from build123d import *

# Parameters (mm, degrees)
SKETCH1_W           = 72
SKETCH1_H           = 47
BOSS_EXTRUDE1_DEPTH = 4
SKETCH3_W           = 72
SKETCH3_H           = 47
SKETCH3_W_2         = 67
SKETCH3_H_2         = 42
BOSS_EXTRUDE3_DEPTH = 32
SKETCH2_R           = 0.9
BOSS_EXTRUDE4_DEPTH = 16
SKETCH4_R           = 2
BOSS_EXTRUDE5_DEPTH = 6
SKETCH5_W           = 12
SKETCH5_H           = 8
CUT_EXTRUDE1_DEPTH  = 6
FILLET2_R           = 2
FILLET3_R           = 2
SKETCH11_W          = 24
SKETCH11_H          = 20
BOSS_EXTRUDE7_DEPTH = 20
SKETCH12_W          = 20
SKETCH12_H          = 16
CUT_EXTRUDE4_DEPTH  = 20
SKETCH13_W          = 15
SKETCH13_H          = 9
CUT_EXTRUDE5_DEPTH  = 20
FILLET4_R           = 2
FILLET5_R           = 2
SKETCH14_W          = 6
SKETCH14_H          = 25
CUT_EXTRUDE6_DEPTH  = 5
FILLET6_R           = 2
SKETCH15_W          = 68
SKETCH15_H          = 6
BOSS_EXTRUDE8_DEPTH = 25
FILLET7_R           = 5
CUT_EXTRUDE7_DEPTH  = 25


with BuildPart() as part:
    # Sketch1 → Boss-Extrude1 (new body)
    with BuildSketch(Plane(origin=(0, 0, 0), x_dir=(1, 0, 0), z_dir=(0, 1, 0))):
        with Locations((25.5, 13)):
            Rectangle(SKETCH1_W, SKETCH1_H)
    extrude(amount=BOSS_EXTRUDE1_DEPTH)

    # Sketch3 → Boss-Extrude3 (add)
    with BuildSketch(Plane(origin=(0, 4, 0), x_dir=(1, 0, 0), z_dir=(0, 1, 0))):
        with Locations((25.5, 13)):
            Rectangle(SKETCH3_W, SKETCH3_H)
        with Locations((25.5, 13)):
            Rectangle(SKETCH3_W_2, SKETCH3_H_2, mode=Mode.SUBTRACT)
    extrude(amount=BOSS_EXTRUDE3_DEPTH)

    # Sketch2 → Boss-Extrude4 (add)
    with BuildSketch(Plane(origin=(0, 4, 0), x_dir=(1, 0, 0), z_dir=(0, 1, 0))):
        with Locations(Location((-1.2, 27.2, 0), (0, 0, 270))):
            Circle(SKETCH2_R)
        with Locations(Location((-1.2, -1.2, 0), (0, 0, 90))):
            Circle(SKETCH2_R)
        with Locations(Location((52.2, -1.2, 0), (0, 0, 270))):
            Circle(SKETCH2_R)
        with Locations(Location((52.2, 27.2, 0), (0, 0, 90))):
            Circle(SKETCH2_R)
    extrude(amount=BOSS_EXTRUDE4_DEPTH)

    # Sketch4 → Boss-Extrude5 (add)
    with BuildSketch(Plane(origin=(0, 4, 0), x_dir=(1, 0, 0), z_dir=(0, 1, 0))):
        with Locations(Location((-1.2, 27.2, 0), (0, 0, 270))):
            Circle(SKETCH4_R)
        with Locations(Location((-1.2, -1.2, 0), (0, 0, 90))):
            Circle(SKETCH4_R)
        with Locations(Location((52.2, -1.2, 0), (0, 0, 270))):
            Circle(SKETCH4_R)
        with Locations(Location((52.2, 27.2, 0), (0, 0, 90))):
            Circle(SKETCH4_R)
    extrude(amount=BOSS_EXTRUDE5_DEPTH)

    # Sketch5 → Cut-Extrude1 (cut)
    with BuildSketch(Plane(origin=(61.5, 0, 0), x_dir=(0, 0, -1), z_dir=(1, 0, 0))):
        with Locations((10, 16)):
            Rectangle(SKETCH5_W, SKETCH5_H)
    extrude(amount=-CUT_EXTRUDE1_DEPTH, mode=Mode.SUBTRACT)

    # Fillet2
    fillet2_edges = [part.edges().sort_by_distance(p)[0] for p in [
        (-10.5, 18, 10.5),
        (-10.5, 18, -36.5),
        (61.5, 18, -36.5),
        (61.5, 18, 10.5),
    ]]
    fillet(fillet2_edges, radius=FILLET2_R)

    # Fillet3
    fillet3_edges = [part.edges().sort_by_distance(p)[0] for p in [
        (60.25, 20, -4),
        (60.25, 20, -16),
    ]]
    fillet(fillet3_edges, radius=FILLET3_R)

    # Sketch11 → Boss-Extrude7 (add)
    with BuildSketch(Plane.ZY.offset(10.5)):
        with Locations((-15.5, 24)):
            Rectangle(SKETCH11_W, SKETCH11_H)
    extrude(amount=BOSS_EXTRUDE7_DEPTH)

    # Sketch12 → Cut-Extrude4 (cut)
    with BuildSketch(Plane(origin=(-8, 0, 0), x_dir=(0, 0, -1), z_dir=(1, 0, 0))):
        with Locations((15.5, 24)):
            Rectangle(SKETCH12_W, SKETCH12_H)
    extrude(amount=-CUT_EXTRUDE4_DEPTH, mode=Mode.SUBTRACT)

    # Sketch13 → Cut-Extrude5 (cut)
    with BuildSketch(Plane.ZY.offset(30.5)):
        with Locations((-15.5, 24)):
            Rectangle(SKETCH13_W, SKETCH13_H)
    extrude(amount=-CUT_EXTRUDE5_DEPTH, mode=Mode.SUBTRACT)

    # Fillet4
    fillet4_edges = [part.edges().sort_by_distance(p)[0] for p in [
        (-18, 16, -25.5),
        (-18, 16, -5.5),
        (-18, 32, -5.5),
        (-18, 32, -25.5),
    ]]
    fillet(fillet4_edges, radius=FILLET4_R)

    # Fillet5
    fillet5_edges = [part.edges().sort_by_distance(p)[0] for p in [
        (-20.5, 34, -27.5),
        (-20.5, 14, -27.5),
        (-20.5, 14, -3.5),
        (-20.5, 34, -3.5),
    ]]
    fillet(fillet5_edges, radius=FILLET5_R)

    # Sketch14 → Cut-Extrude6 (cut)
    with BuildSketch(Plane.ZY.offset(10.5)):
        with Locations((3, 24.5)):
            Rectangle(SKETCH14_W, SKETCH14_H)
    extrude(amount=-CUT_EXTRUDE6_DEPTH, mode=Mode.SUBTRACT)

    # Fillet6
    fillet6_edges = [part.edges().sort_by_distance(p)[0] for p in [
        (-9.25, 12, 0),
        (-9.25, 12, 6),
    ]]
    fillet(fillet6_edges, radius=FILLET6_R)

    # Sketch15 → Boss-Extrude8 (add)
    with BuildSketch(Plane.XY.offset(10.5)):
        with Locations((25.5, 3)):
            Rectangle(SKETCH15_W, SKETCH15_H)
    extrude(amount=BOSS_EXTRUDE8_DEPTH)

    # Fillet7
    fillet7_edges = [part.edges().sort_by_distance(p)[0] for p in [
        (-8.5, 3, 35.5),
        (59.5, 3, 35.5),
    ]]
    fillet(fillet7_edges, radius=FILLET7_R)

    # Sketch16 → Cut-Extrude7 (cut)
    with BuildSketch(Plane(origin=(0, 6, 0), x_dir=(1, 0, 0), z_dir=(0, 1, 0))):
        with BuildLine():
            Line((5.870048695, -18.078882232), (45.129951305, -18.078882232))
            ThreePointArc((45.129951305, -18.078882232), (49.279951305, -22.228882232), (45.129951305, -26.378882232))
            Line((45.129951305, -26.378882232), (5.870048695, -26.378882232))
            ThreePointArc((5.870048695, -26.378882232), (1.720048695, -22.228882232), (5.870048695, -18.078882232))
        make_face()
    extrude(amount=-CUT_EXTRUDE7_DEPTH, mode=Mode.SUBTRACT)


solid = part.part
Could you check a few things on this model? Use its own coordinates, in mm. A direction names the side the tool comes from. Coordinates: 2 decimals unless noted, no trailing zeros. Order: outer loops, then holes, each group sorted by start corner. A loop starts at its lowest first (then second) coordinate and runs counter-clockwise, first axis right, second up.
Q1. Suppose I cut it at C-C on x = 25. Please give me the cut outline in (y, z).
Q2. Will these pins go through, and if not, where does the flat tip stop? pin 1 (1 mm diameter, centred on x = -2, y = 18, fed in from +Z); pin 2 (3 mm diameter, centred on x = 52.5, z = 1, fed in from +Y); pin 3 (2 mm diameter, centred on x = -8.5, z = 3.5, fed in from +Y).
Q3. Suppose I cut it at A-A on y = 9. Please give me the cut outline in (x, z).
Q4. Thinking about a two-plate mould opening in Z: for faces 1 (the flat face through (-30.5, 29, -16)), 2 (the cylindrical face through (60.9, 17.75, -35.93)), 3 (the flat face through (-18, 24, -5.5)), 4 (the flat face through (25, 3, 35.5)), which applies, released by +Z, released by -Z, zero draft, split by the parting line, or undercut?
Q5. Please list where these lines run through material, in increasing order: L1, parallel to X at y = 22, z = -28; L2, parallel to Z at x = 25, y = 26.5; L3, parallel to Z at x = 45, y = 3.5.
Q6. Suppose I cut it at B-B on y = 23. Please give me the cut outline in (x, z), and give its area (3 significant figures).
Q7. Suppose I cut it at D-D on z = 7. Please give me the cut outline in (x, y), and give its area (3 significant figures).
Q8. Which directions (+Z, -Z, +X, -X, +Y, -Y) give clear straight access to the entire face, cutting with the end or side of a thin tool? Please do faces 5 (the flat face through (-20, 24, -3.5)), 6 (the flat face through (-9, 25, 0)), 7 (the flat face through (-8, 13, -17)), 8 (the cylindrical face through (1.72, 3.04, 22.32)).
Answer:
1. outline: (0, -36.5) - (36, -36.5) - (36, -34) - (4, -34) - (4, 8) - (36, 8) - (36, 10.5) - (6, 10.5) - (6, 18.08) - (0, 18.08) - close; (0, 26.38) - (6, 26.38) - (6, 35.5) - (0, 35.5) - close
2. pin 1: stops at z = 10.5
2. pin 2: stops at y = 20
2. pin 3: stops at y = 12.06
3. outline: (-10.5, -34.5) arc R2 ccw to (-8.5, -36.5) - (59.5, -36.5) arc R2 ccw to (61.5, -34.5) - (61.5, 8.5) arc R2 ccw to (59.5, 10.5) - (-8.5, 10.5) arc R2 ccw to (-10.5, 8.5) - close; circle Ø4 at (-1.2, -27.2); circle Ø4 at (-1.2, 1.2); circle Ø4 at (52.2, -27.2); circle Ø4 at (52.2, 1.2); hole (-8, -34) - (59, -34) - (59, 8) - (-8, 8) - close
4. face 1: zero draft
4. face 2: released by -Z
4. face 3: undercut
4. face 4: released by +Z
5. L1: x = -10.5 to -8, 59 to 61.5
5. L2: z = -36.5 to -34, 8 to 10.5
5. L3: z = -36.5 to 18.08, 26.38 to 35.5
6. outline: (-30.5, -27.5) - (-10.5, -27.5) - (-10.5, -34.5) arc R2 ccw to (-8.5, -36.5) - (59.5, -36.5) arc R2 ccw to (61.5, -34.5) - (61.5, 8.5) arc R2 ccw to (59.5, 10.5) - (-8.5, 10.5) arc R2 ccw to (-10.5, 8.5) - (-10.5, 6) - (-8, 6) - (-8, 8) - (59, 8) - (59, -34) - (-8, -34) - (-8, -25.5) - (-28, -25.5) - (-28, -23) - (-30.5, -23) - close; (-30.5, -8) - (-28, -8) - (-28, -5.5) - (-8, -5.5) - (-8, 0) - (-10.5, 0) - (-10.5, -3.5) - (-30.5, -3.5) - close
6. area: 594 mm2
7. outline: (-10.5, 0) - (61.5, 0) - (61.5, 36) - (59, 36) - (59, 4) - (-8, 4) - (-8, 36) - (-10.5, 36) - close
7. area: 448 mm2
8. face 5: +Z, -X, +Y, -Y
8. face 6: -X, +Y
8. face 7: +Y
8. face 8: +Y, -Y
